Read the model definition and answer for the solid it produces. Units are mm, in the model's axes. Face numbers are marked on the shaded views. A direction names the side the tool comes from. Round coordinates to 2 decimals unless told otherwise and drop trailing zeros. Loops run counter-clockwise (first coordinate to the right, second up) from the corner with the lowest first, then second, coordinate; pieces in that order, holes last. Notation, with made-up numbers: (-31.5, -37) - (0.5, -37) arc R16 cw to (0.5, -18) - close; hole circle Ø4 at (-7, 25). An arc over 180 degrees is marked (long way). Answer as CSV lines item,"result".
```python
from build123d import *

# Parameters (mm, degrees)
SKETCH1_W           = 100
SKETCH1_H           = 100
BOSS_EXTRUDE1_DEPTH = 60
SKETCH2_W           = 98
SKETCH2_H           = 98
CUT_EXTRUDE1_DEPTH  = 225
SKETCH3_R           = 1
CUT_EXTRUDE2_DEPTH  = 118
FILLET1_R           = 1


with BuildPart() as part:
    # Sketch1 → Boss-Extrude1 (new body)
    with BuildSketch(Plane(origin=(0, 0, 0), x_dir=(1, 0, 0), z_dir=(0, 1, 0))):
        Rectangle(SKETCH1_W, SKETCH1_H)
    extrude(amount=BOSS_EXTRUDE1_DEPTH)

    # Sketch2 → Cut-Extrude1 (cut)
    with BuildSketch(Plane(origin=(0, 60, 0), x_dir=(1, 0, 0), z_dir=(0, 1, 0))):
        Rectangle(SKETCH2_W, SKETCH2_H)
    extrude(amount=-CUT_EXTRUDE1_DEPTH, mode=Mode.SUBTRACT)

    # Sketch3 → Cut-Extrude2 (cut)
    with BuildSketch(Plane.ZY.offset(50)):
        with BuildLine():
            ThreePointArc((-26, 55), (-25, 54), (-24, 55))
            Line((-24, 55), (-26, 55))
        make_face()
        with BuildLine():
            Line((-26, 55), (-24, 55))
            ThreePointArc((-24, 55), (-25, 56), (-26, 55))
        make_face()
        with Locations((25, 55)):
            Circle(SKETCH3_R)
    extrude(amount=-CUT_EXTRUDE2_DEPTH, mode=Mode.SUBTRACT)

    # Fillet1
    fillet1_edges = [part.edges().sort_by_distance(p)[0] for p in [
        (50, 30, 50),
        (-50, 30, 50),
        (-50, 30, -50),
        (50, 30, -50),
    ]]
    fillet(fillet1_edges, radius=FILLET1_R)


solid = part.part
```
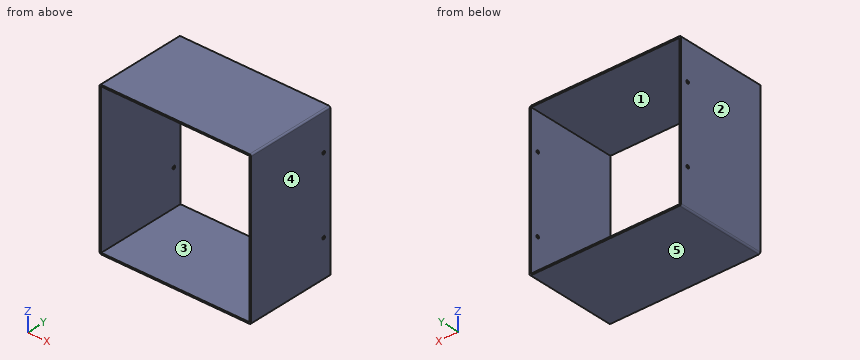
1) A cutting plane is placed at C-C, the plane y = 49. Determine the outline of the cut face in (x, z).
Entries:
outline,"(-50, -49) arc R1 ccw to (-49, -50) - (49, -50) arc R1 ccw to (50, -49) - (50, 49) arc R1 ccw to (49, 50) - (-49, 50) arc R1 ccw to (-50, 49) - close; hole (-49, -49) - (49, -49) - (49, 49) - (-49, 49) - close"
2) A tool of negligible diameter and unlimited length cuts with its end or side. For the marked faces 1 and 2, from which of +Z, -Z, +X, -X, +Y, -Y can it reach the whole face along a straight path? Write none if from no direction.
Entries:
face 1,"+Y, -Y"
face 2,"+Z, -Z, -X, +Y, -Y"
3) Find the intervals of material crossed by line 1 (Z direction, x = -41, y = 4.5); line 2 (Y direction, x = -49.3, z = 25), in increasing order.
Entries:
line 1,"z = -50 to -49, 49 to 50"
line 2,"y = 0 to 54, 56 to 60"
4) A cutting plane is placed at A-A, the plane x = 16.5. Determine the outline of the cut face in (y, z), plus the area to 3 significant figures.
Entries:
outline,"(0, -50) - (60, -50) - (60, -49) - (0, -49) - close; (0, 49) - (60, 49) - (60, 50) - (0, 50) - close"
area,"120 mm^2"
5) A cutting plane is placed at B-B, the plane z = 41. Determine the outline of the cut face in (x, y), plus the area to 3 significant figures.
Entries:
outline,"(-50, 0) - (-49, 0) - (-49, 60) - (-50, 60) - close; (49, 0) - (50, 0) - (50, 60) - (49, 60) - close"
area,"120 mm^2"
6) The mould has two halves that part along Z. Classify the marked faces 3, 4 and 5: pulls with the +Z half, pulls with the -Z half, needs draft (parallel to the pull), parting line crosses it, or undercut.
Entries:
face 3,"undercut"
face 4,"needs draft"
face 5,"pulls with the -Z half"
